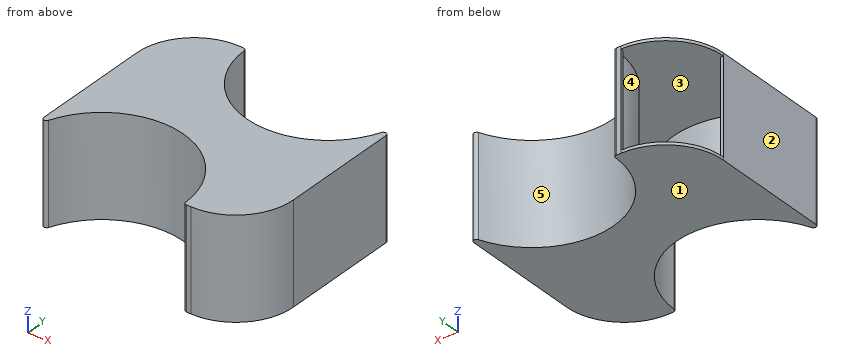
from build123d import *

# Parameters (mm, degrees)
EXTRUDE_1_DEPTH = 35
FILLET_1_R      = 1
FILLET_2_R      = 20
SHELL_START     = 1
SHELL_4_DEPTH   = 33


# Read off the part's stored shape, not the designer's step: 抽壳4
with BuildPart() as part:
    # 草图3 → 凸台-拉伸1 (new body)
    with BuildSketch(Plane.XY):
        with BuildLine():
            Line((-28.5, 0), (-51.03000000000027, -2.76e-15))
            Line((-51.03000000000027, -2.76e-15), (-51.029999999999994, -72))
            ThreePointArc((-51.029999999999994, -72), (-22.529999999999987, -43.5), (5.970000000000013, -72))
            Line((5.970000000000013, -72), (28.5, -72))
            Line((28.5, -72), (28.5, 0))
            ThreePointArc((28.5, 0), (-5.24e-15, -28.5), (-28.5, 0))
        make_face()
    extrude(amount=EXTRUDE_1_DEPTH)

    # 圆角1
    fillet_1_edges = [part.edges().sort_by_distance(p)[0] for p in [
        (5.970000000000011, -72, 17.5),
        (-51.02999999999999, -72, 17.5),
        (-28.5, -2.63e-15, 17.5),
    ]]
    fillet(fillet_1_edges, radius=FILLET_1_R)
    fillet_1_2_edges = [part.edges().sort_by_distance(p)[0] for p in [
        (28.5, 0, 17.5),
    ]]
    fillet(fillet_1_2_edges, radius=FILLET_1_R)

    # 圆角2
    fillet_2_edges = [part.edges().sort_by_distance(p)[0] for p in [
        (28.5, -72, 17.5),
        (-51.03000000000027, -2.76e-15, 17.5),
    ]]
    fillet(fillet_2_edges, radius=FILLET_2_R)

    # 抽壳4 outline → 抽壳4 (cut)
    with BuildSketch(Plane.XY.offset(SHELL_START)):
        with BuildLine():
            Line((-51.03, -20), (-50.03, -20))
            Line((-50.03, -20), (-50.03, -61.322921748))
            ThreePointArc((-50.03, -61.322921748), (-17.59091317, -42.916406321), (6.953045976, -71))
            Line((6.953045976, -71), (8.5, -71))
            ThreePointArc((8.5, -71), (21.935028843, -65.435028843), (27.5, -52))
            Line((27.5, -52), (27.5, -10.677078252))
            ThreePointArc((27.5, -10.677078252), (-4.93908683, -29.083593679), (-29.483045976, -1))
            Line((-29.483045976, -1), (-31.03, -1))
            Line((-31.03, -1), (-31.03, 0))
            ThreePointArc((-31.03, 0), (-45.172135624, -5.857864376), (-51.03, -20))
        make_face()
    extrude(amount=SHELL_4_DEPTH, mode=Mode.SUBTRACT)


solid = part.part
Design review of the part built by this model. Coordinates are the model's own, in mm. Face numbers are marked on the shaded views. A direction names the side the tool comes from. Coordinates: 2 decimals unless noted, no trailing zeros. Order: outer loops, then holes, each group sorted by start corner. A loop starts at its lowest first (then second) coordinate and runs counter-clockwise, first axis right, second up.
Item 1: Take a section at D-D, the plane y = -59.5. Write out the cut boundary in (x, z).
Item 2: For pin 1 Ø1.7 at (x, z) = (7.5, 14) entering from +Y; pin 2 Ø3 at (x, z) = (-38.5, 13) entering from +Y; pin 3 Ø4 at (x, z) = (9.5, 18.5) entering from +Y, all flat-tipped, find the tip position at first contact; note any pin that passes through.
Item 3: For the marked faces 4 and 5, list the 3-axis set-ups (+Z, -Z, +X, -X, +Y, -Y) from which the entire face can be reached by the end or side of a thin tool; tool diameter is ignored.
Item 4: For line 1 (Z direction, x = 16, y = -39.5); line 2 (X direction, y = -54, z = 33.5); line 3 (X direction, y = -34.5, z = 33), list the stretches that pass through material, from the lowest coordinate up.
Item 5: Take a section at C-C, the plane x = 23.5. Write out the cut boundary in (y, z), then the cut area to 3 significant figures.
Item 6: Take a section at A-A, the plane y = -12.5. Write out the cut boundary in (x, z), then the cut area to 3 significant figures.
Item 7: The part is to be moulded in two halves that separate along Z. For the marked faces 1, 2 and 3, say which applies: pulls with the +Z half, pulls with the -Z half, needs draft (parallel to the pull), parting line crosses it, or undercut.
Item 8: Take a section at B-B, the plane y = -39.5. Write out the cut boundary in (x, z), then the cut area to 3 significant figures.
The answers:
1. outline: (-51.03, 0) - (-48.14, 0) - (-48.14, 35) - (-51.03, 35) - close; (3.08, 0) - (27.04, 0) - (27.04, 35) - (3.08, 35) - close; hole (-50.03, 1) - (-49.25, 1) - (-49.25, 34) - (-50.03, 34) - close; hole (4.19, 1) - (25.96, 1) - (25.96, 34) - (4.19, 34) - close
2. pin 1: stops at y = -27.25
2. pin 2: stops at y = -46.29
2. pin 3: stops at y = -26.08
3. face 4: none
3. face 5: +Z, -Z, +Y
4. line 1: z = 0 to 1, 34 to 35
4. line 2: x = -51.03 to -50.03, -45.9 to -44.63, -0.43 to 0.84, 27.39 to 28.4
4. line 3: x = -51.03 to -50.03, 27.5 to 28.5
5. outline: (-65.23, 0) - (-16.12, 0) - (-16.12, 35) - (-65.23, 35) - close; hole (-63.66, 1) - (-17.83, 1) - (-17.83, 34) - (-63.66, 34) - close
5. area: 206 mm2
6. outline: (-49.57, 0) - (-25.61, 0) - (-25.61, 35) - (-49.57, 35) - (-49.57, 34) - (-26.72, 34) - (-26.72, 1) - (-49.57, 1) - close; (25.61, 0) - (28.5, 0) - (28.5, 35) - (25.61, 35) - close; hole (26.72, 1) - (27.5, 1) - (27.5, 34) - (26.72, 34) - close
6. area: 160 mm2
7. face 1: pulls with the -Z half
7. face 2: needs draft
7. face 3: undercut
8. outline: (-51.03, 0) - (28.5, 0) - (28.5, 35) - (-51.03, 35) - close; hole (-50.03, 1) - (27.5, 1) - (27.5, 34) - (-50.03, 34) - close
8. area: 225 mm2
